Autodesk Inventor part; units mm, degrees
ref_plane "YZ Plane" through (0, 0, 0) normal (1, 0, 0) x (0, 1, 0)
ref_plane "XZ Plane" through (0, 0, 0) normal (0, 1, 0) x (-1, 0, 0)
ref_plane "XY Plane" through (0, 0, 0) normal (0, 0, 1) x (1, 0, 0)
sketch "Sketch1" plane through (0, 0, 0) normal (0, 1, 0) x (-1, 0, 0)
  line L0 (-25.4, -25.4) -> (25.4, -25.4)
  line L1 (25.4, -25.4) -> (25.4, 25.4)
  line L2 (25.4, 25.4) -> (-25.4, 25.4)
  line L3 (-25.4, 25.4) -> (-25.4, -25.4)
  line L4 (-25.4, -25.4) -> (25.4, 25.4) construction
  line L5 (25.4, -25.4) -> (-25.4, 25.4) construction
  line L6 (-15.875, 15.875) -> (15.875, 15.875)
  line L7 (15.875, 15.875) -> (15.875, -15.875)
  line L8 (15.875, -15.875) -> (-15.875, -15.875)
  line L9 (-15.875, -15.875) -> (-15.875, 15.875)
  line L10 (-15.875, 15.875) -> (15.875, -15.875) construction
  line L11 (15.875, 15.875) -> (-15.875, -15.875) construction
  circle A0 centre (15.875, 15.875) radius 2.5
  circle A1 centre (15.875, -15.875) radius 2.5
  circle A2 centre (-15.875, -15.875) radius 2.5
  circle A3 centre (-15.875, 15.875) radius 2.5
  point P0 (0, 0)
  dimension "d0" = 50.8
  dimension "d1" = 50.8
  dimension "d2" = 31.75
  dimension "d3" = 31.75
  dimension "d4" = 5
  dimension "d5" = 5
  dimension "d6" = 5
  dimension "d7" = 5
extrude "Extrusion1" add sketch "Sketch1" along normal blind 2.54 contours L3 L2 L1 L0 | L6 A0 L7 A1 L8 A2 L9 A3
properties part number "l channel guide"
The model under review builds one solid part; all positions refer to its coordinate system, in mm. Round coordinates to 2 decimals unless told otherwise and drop trailing zeros. Order: outer loops, then holes, each group sorted by start corner. A loop starts at its lowest first (then second) coordinate and runs counter-clockwise, first axis right, second up.
Item 1: Draft analysis for pull direction X (two halves, no side actions). For faces 1 (the flat face through (25.4, 1, 0)), 2 (the cylindrical face through (-13.377, 1.252, -15.985)), 3 (the flat face through (0, 1, 25.4)), 4 (the flat face through (-25.4, 1, 0)), state which applies: released by +X, released by -X, zero draft, split by the parting line, or undercut.
Working result:
face 1: released by +X
face 2: undercut
face 3: zero draft
face 4: released by -X
Item 2: Add section A-A, the plane z = 16.5. State the section outline as (x, y) points.
Working result:
outline: (-25.4, 0) - (-18.3, 0) - (-18.3, 2.54) - (-25.4, 2.54) - close; (-13.45, 0) - (13.45, 0) - (13.45, 2.54) - (-13.45, 2.54) - close; (18.3, 0) - (25.4, 0) - (25.4, 2.54) - (18.3, 2.54) - close
Item 3: Add section C-C, the plane x = 14. State the section outline as (y, z) points.
Working result:
outline: (0, -25.4) - (2.54, -25.4) - (2.54, -17.53) - (0, -17.53) - close; (0, -14.22) - (2.54, -14.22) - (2.54, 14.22) - (0, 14.22) - close; (0, 17.53) - (2.54, 17.53) - (2.54, 25.4) - (0, 25.4) - close
Item 4: To check wall thickness, follow probe 1 along X at (y, z) = (0.3, -17); probe 2 along X at (y, z) = (1.9, -15); probe 3 along Z at (x, y) = (-16.5, 0.25). State the ranges of each line that lie inside material, in increasing order.
Working result:
probe 1: x = -25.4 to -18.11, -13.64 to 13.64, 18.11 to 25.4
probe 2: x = -25.4 to -18.22, -13.53 to 13.53, 18.22 to 25.4
probe 3: z = -25.4 to -18.3, -13.45 to 13.45, 18.3 to 25.4
Item 5: Add section B-B, the plane y = 0.95. State the section outline as (x, z) points (3 decimals), and give its area (3 significant figures).
Working result:
outline: (-25.4, -25.4) - (25.4, -25.4) - (25.4, 25.4) - (-25.4, 25.4) - close; hole circle Ø5 at (-15.875, -15.875); hole circle Ø5 at (-15.875, 15.875); hole circle Ø5 at (15.875, -15.875); hole circle Ø5 at (15.875, 15.875)
area: 2,500 mm2
